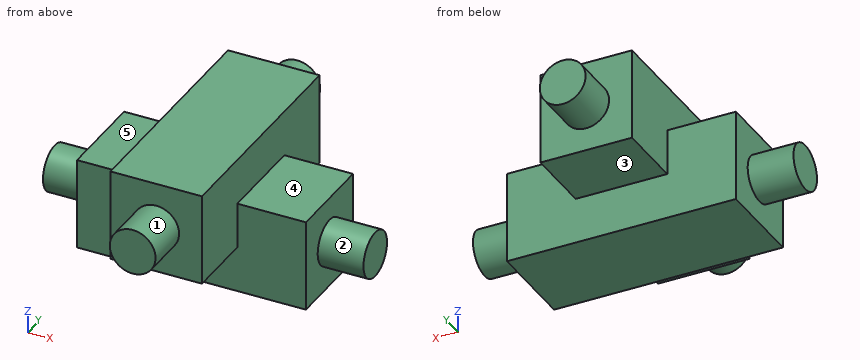
```python
from build123d import *

# Parameters (mm, degrees)
SKETCH1_W           = 20
SKETCH1_H           = 20
BOSS_EXTRUDE1_DEPTH = 25
SKETCH2_W           = 20
SKETCH2_H           = 20
BOSS_EXTRUDE2_DEPTH = 25
SKETCH3_R           = 5
BOSS_EXTRUDE3_DEPTH = 35
SKETCH5_R           = 5
BOSS_EXTRUDE4_DEPTH = 35


with BuildPart() as part:
    # Sketch1 → Boss-Extrude1 (new, symmetric)
    with BuildSketch(Plane(origin=(0, 0, 0), x_dir=(1, 0, 0), z_dir=(0, 1, 0))):
        Rectangle(SKETCH1_W, SKETCH1_H)
    extrude(amount=BOSS_EXTRUDE1_DEPTH, both=True)

    # Sketch2 → Boss-Extrude2 (add, symmetric)
    with BuildSketch(Plane(origin=(0, 0, 0), x_dir=(0, 0, -1), z_dir=(1, 0, 0))):
        with Locations((10, 0)):
            Rectangle(SKETCH2_W, SKETCH2_H)
    extrude(amount=BOSS_EXTRUDE2_DEPTH, both=True)

    # Sketch3 → Boss-Extrude3 (add, symmetric)
    with BuildSketch(Plane(origin=(0, 0, 0), x_dir=(1, 0, 0), z_dir=(0, 1, 0))):
        with Locations(Location((0, 0, 0), (0, 0, 270))):
            Circle(SKETCH3_R)
    extrude(amount=BOSS_EXTRUDE3_DEPTH, both=True)

    # Sketch5 → Boss-Extrude4 (add, symmetric)
    with BuildSketch(Plane(origin=(0, 0, 0), x_dir=(0, 0, -1), z_dir=(1, 0, 0))):
        with Locations((10, 0)):
            Circle(SKETCH5_R)
    extrude(amount=BOSS_EXTRUDE4_DEPTH, both=True)


solid = part.part
```
Geometry check sheet. Reference: the model listing, model coordinates, mm. Face numbers are marked on the shaded views. A direction names the side the tool comes from. Coordinates: 2 decimals unless noted, no trailing zeros. Order: outer loops, then holes, each group sorted by start corner. A loop starts at its lowest first (then second) coordinate and runs counter-clockwise, first axis right, second up.
Item 1: Scan lines: line 1 along Y through (x, z) = (-4, 7.5); line 2 along Z through (x, y) = (-6, 15). Record each from-to range of solid material in increasing order.
Item 2: Section check C-C (z = -1.75). Enter the section's corners in (x, y), plus the area to 3 significant figures.
Item 3: Depth check by flat-ended pin: pin 1 (1.5 mm diameter, centred on y = -12.5, z = -15.5, fed in from -X); pin 2 (6 mm diameter, centred on x = -12, z = -16.5, fed in from -Y); pin 3 (12 mm diameter, centred on x = 16.5, y = -3, fed in from +Z); pin 4 (1.5 mm diameter, centred on y = 8.5, z = -1, fed in from +X). Enter the tip coordinate at first touch or a pass-through.
Item 4: Section check D-D (x = 9). Enter the section's corners in (y, z).
Item 5: Tool access check on the marked faces 1, 2, 3, 4 and 5. Record the directions out of +Z, -Z, +X, -X, +Y, -Y that give a thin tool (end or side, any length) a straight path to the whole face; none if there is none.
Item 6: Section check B-B (y = 0). Enter the section's corners in (x, z), plus the area to 3 significant figures.
Item 7: Section check A-A (x = 0). Enter the section's corners in (y, z), plus the area to 3 significant figures.
Check sheet entries:
1. line 1: y = -25 to 25
1. line 2: z = -10 to 10
2. outline: (-25, -10) - (-10, -10) - (-10, -25) - (-4.68, -25) - (-4.68, -35) - (4.68, -35) - (4.68, -25) - (10, -25) - (10, -10) - (25, -10) - (25, 10) - (10, 10) - (10, 25) - (4.68, 25) - (4.68, 35) - (-4.68, 35) - (-4.68, 25) - (-10, 25) - (-10, 10) - (-25, 10) - close
2. area: 1,790 mm2
3. pin 1: passes through
3. pin 2: stops at y = -10
3. pin 3: stops at z = 0
3. pin 4: stops at x = 25
4. outline: (-25, -10) - (-10, -10) - (-10, -20) - (10, -20) - (10, -10) - (25, -10) - (25, 10) - (-25, 10) - close
5. face 1: -Y
5. face 2: +X
5. face 3: -Z, +X, -X, +Y
5. face 4: +Z, +X, +Y, -Y
5. face 5: +Z, -X, +Y, -Y
6. outline: (-35, -15) - (-25, -15) - (-25, -20) - (25, -20) - (25, -15) - (35, -15) - (35, -5) - (25, -5) - (25, 0) - (10, 0) - (10, 10) - (-10, 10) - (-10, 0) - (-25, 0) - (-25, -5) - (-35, -5) - close
6. area: 1,400 mm2
7. outline: (-35, -5) - (-25, -5) - (-25, -10) - (-10, -10) - (-10, -20) - (10, -20) - (10, -10) - (25, -10) - (25, -5) - (35, -5) - (35, 5) - (25, 5) - (25, 10) - (-25, 10) - (-25, 5) - (-35, 5) - close
7. area: 1,400 mm2
